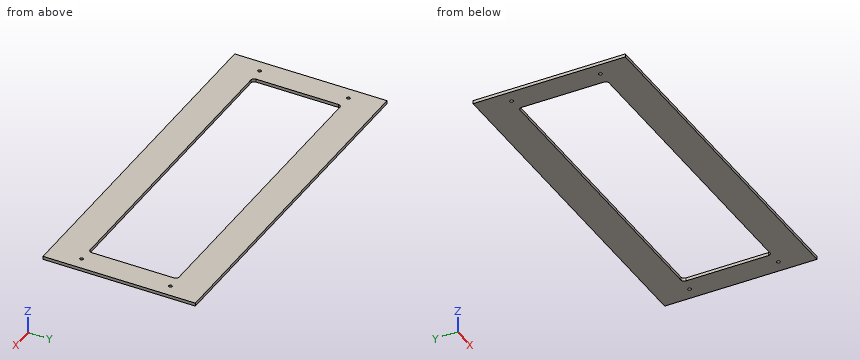
Autodesk Inventor part; units mm, degrees
ref_plane "YZ Plane" through (0, 0, 0) normal (1, 0, 0) x (0, 1, 0)
ref_plane "XZ Plane" through (0, 0, 0) normal (0, 1, 0) x (-1, 0, 0)
ref_plane "XY Plane" through (0, 0, 0) normal (0, 0, 1) x (1, 0, 0)
sketch "Sketch1" plane through (0, 0, 0) normal (0, 0, 1) x (1, 0, 0)
  line L0 (0, 0) -> (355.6, 0)
  line L1 (355.6, 0) -> (355.6, 152.4)
  line L2 (355.6, 152.4) -> (0, 152.4)
  line L3 (0, 152.4) -> (0, 0)
  dimension "d0" = 152.4
  dimension "d1" = 355.6
extrude "Extrusion1" add sketch "Sketch1" along normal blind 3.175
sketch "Sketch2" plane through (0, 0, 3.175) normal (0, 0, 1) x (1, 0, 0)
  line L0 (355.6, 0) -> (355.6, 152.4)
  line L1 (0, 152.4) -> (0, 0)
  line L2 (355.6, 152.4) -> (0, 152.4)
  line L3 (0, 0) -> (355.6, 0)
  point P0 (12.7, 31.75)
  point P1 (12.7, 120.65)
  point P2 (342.9, 120.65)
  point P3 (342.9, 31.75)
  dimension "d4" = 12.7
  dimension "d5" = 12.7
  dimension "d6" = 12.7
  dimension "d7" = 12.7
  dimension "d8" = 31.75
  dimension "d9" = 31.75
  dimension "d10" = 31.75
  dimension "d11" = 31.75
hole "Hole1" at (12.7, 31.75, 3.175) at (12.7, 120.65, 3.175) at (342.9, 120.65, 3.175) at (342.9, 31.75, 3.175) direction (0, 0, -1) diameter 3.302 end through all
sketch "Sketch3" plane through (0, 0, 3.175) normal (0, 0, 1) x (1, 0, 0)
  line L0 (25.4, 31.75) -> (330.2, 31.75)
  line L1 (330.2, 31.75) -> (330.2, 120.65)
  line L2 (330.2, 120.65) -> (25.4, 120.65)
  line L3 (25.4, 120.65) -> (25.4, 31.75)
  line L4 (0, 152.4) -> (0, 0)
  circle A0 centre (342.9, 120.65) radius 1.651
  circle A1 centre (12.7, 31.75) radius 1.651
  circle A2 centre (12.7, 120.65) radius 1.651
  circle A3 centre (342.9, 31.75) radius 1.651
  line L5 (0, 0) -> (355.6, 0)
  line L6 (355.6, 0) -> (355.6, 152.4)
  line L7 (355.6, 152.4) -> (0, 152.4)
  line L8 (0, 152.4) -> (0, 0)
  dimension "d27" = 25.4
  dimension "d28" = 304.8
  dimension "d29" = 31.75
  dimension "d30" = 88.9
extrude "Extrusion2" cut sketch "Sketch3" against normal blind 3.175 contours L3 L2 L1 L0
fillet "Fillet1" radius 3.175 4 edges at (25.4, 31.75, 1.5875) (25.4, 120.65, 1.5875) (330.2, 120.65, 1.5875) (330.2, 31.75, 1.5875)
properties part number "LFEV2017_TSI_003"
Part model, mm, in its own coordinate system. Round coordinates to 2 decimals unless told otherwise and drop trailing zeros. Write each loop counter-clockwise with the first axis right and the second up, starting at its lowest first coordinate (ties: lowest second). Pieces come first, ordered by that corner, then holes. Notation, with made-up numbers: M 13.25,8 L 36.25,8 A19 cw 36.25,26 Z; hole C 67.5,15 d10. An arc over 180 degrees is marked long. Answer as CSV lines item,"result". Start each with the question number.
1) Drop flat-ended pins along their axis: pin 1 (1 mm diameter, centred on y = 82, z = 1.5, fed in from -X); pin 2 (2.5 mm diameter, centred on x = 12.7, y = 120.65, fed in from -Z). Give the stop position or say it passes through.
2) Band-saw the part on C-C (z = 1.15). List the corners of the cut face in (x, y) (3 decimals).
3) Band-saw the part on B-B (x = 106.5). List the corners of the cut face in (y, z) (3 decimals), then the cut area to 3 significant figures.
4) Drill centre lines: L1, parallel to Y at x = 12.7, z = 2.3; L2, parallel to Y at x = 314.5, z = 2.1; L3, parallel to X at y = 62, z = 2.75. Where is each one in solid material? Low to high.
5) Band-saw the part on A-A (y = 113). List the corners of the cut face in (x, z) (3 decimals).
Worked out:
1,pin 1,"x = 0"
1,pin 2,"through"
2,outline,"M 0,0 L 355.6,0 L 355.6,152.4 L 0,152.4 Z; hole C 12.7,31.75 d3.302; hole C 12.7,120.65 d3.302; hole M 25.4,34.925 A3.175 ccw 28.575,31.75 L 327.025,31.75 A3.175 ccw 330.2,34.925 L 330.2,117.475 A3.175 ccw 327.025,120.65 L 28.575,120.65 A3.175 ccw 25.4,117.475 Z; hole C 342.9,31.75 d3.302; hole C 342.9,120.65 d3.302"
3,outline,"M 0,0 L 31.75,0 L 31.75,3.175 L 0,3.175 Z; M 120.65,0 L 152.4,0 L 152.4,3.175 L 120.65,3.175 Z"
3,area,"202 mm²"
4,L1,"0 to 30.1, 33.4 to 119, 122.3 to 152.4"
4,L2,"0 to 31.75, 120.65 to 152.4"
4,L3,"0 to 25.4, 330.2 to 355.6"
5,outline,"M 0,0 L 25.4,0 L 25.4,3.175 L 0,3.175 Z; M 330.2,0 L 355.6,0 L 355.6,3.175 L 330.2,3.175 Z"
